Autodesk Inventor part; units mm, degrees
ref_plane "工作平面1" through (0, 0, 5.8) normal (0, 0, 1) x (1, 0, 0)
ref_plane "YZ Plane" through (0, 0, 0) normal (1, 0, 0) x (0, 1, 0)
ref_plane "XZ Plane" through (0, 0, 0) normal (0, 1, 0) x (-1, 0, 0)
sketch "草圖1" plane through (0, 0, 0) normal (0, 0, 1) x (1, 0, 0)
  circle A0 centre (0, 0) radius 26
  dimension "d0" = 52
extrude "擠出1" add sketch "草圖1" along normal blind 12.2
sketch "草圖2" plane through (0, 0, 12.2) normal (0, 0, 1) x (1, 0, 0)
  circle A0 centre (0, 0) radius 26
  circle A1 centre (0, 0) radius 20
  dimension "d3" = 40
extrude "擠出2" cut sketch "草圖2" against normal through all contours A1
sketch "草圖3" plane through (0, 0, 0) normal (0, 0, -1) x (-1, 0, 0)
  circle A0 centre (0, 0) radius 20
  circle A1 centre (0, 0) radius 26
  circle A2 centre (0, 0) radius 22.45
  dimension "d6" = 44.9
extrude "擠出3" cut sketch "草圖3" against normal blind 8.2 contours A2
ref_plane "工作平面1" through (0, 0, 5.8) normal (0, 0, 1) x (1, 0, 0)
sketch "草圖4" plane through (0, 0, 5.8) normal (0, 0, 1) x (1, 0, 0)
  circle A0 centre (0, 0) radius 24.4
  circle A1 centre (0, 0) radius 26
  dimension "d10" = 48.8
extrude "擠出4" cut sketch "草圖4" against normal blind 2.8
chamfer "倒角1" distance 0.4 angle 45 3 edges at (-26, 0, 12.2) (-26, 0, 0) (22.45, 0, 0)
chamfer "倒角2" distance 0.3 angle 45 2 edges at (-20, 0, 8.2) (-20, 0, 12.2)
properties part number "鑄鐵SLEEVE"
Check sheet for the modelled part. Datum: model origin and axes. Units: mm. A direction names the side the tool comes from. Round coordinates to 2 decimals unless told otherwise and drop trailing zeros. Write each loop counter-clockwise with the first axis right and the second up, starting at its lowest first coordinate (ties: lowest second). Pieces come first, ordered by that corner, then holes. Notation, with made-up numbers: (73.5, 86.25) -> (98.5, 86.25) arc R14 cw to (98.5, 92.25) -> close; hole circle Ø3 at (69.5, -38). An arc over 180 degrees is marked (long way). Put each result on its own line as item: value.
(1) Tool access check on faces 1 (the face through (-4.336, -19.524, 10.224)), 2 (the face through (-24.376, 1.073, 4.42)). Record the directions out of +Z, -Z, +X, -X, +Y, -Y that give a thin tool (end or side, any length) a straight path to the whole face; none if there is none.
Values found:
face 1: +Z, -Z
face 2: none
(2) Sectioned sample at D-D (z = 10.5). Enter the section's corners in (x, y).
Values found:
outline: circle Ø52 at (0, 0); hole circle Ø40 at (0, 0)
(3) Go/stop test with flat-tipped pins: pin 1 Ø10 at (x, y) = (6.5, -20.5) entering from -Z; pin 2 Ø4 at (x, z) = (-14.5, 9.5) entering from -Y; pin 3 Ø1 at (x, z) = (-11, 8) entering from -Y; pin 4 Ø6 at (y, z) = (-10, 6) entering from -X. Record where each tip stops, or that it passes through.
Values found:
pin 1: stops at z = 0
pin 2: stops at y = -22.8
pin 3: stops at y = -23.79
pin 4: stops at x = -25.04
(4) Mould release check, pull along X, two halves, no side actions. Record for faces 3 (the face through (17, -12, 8.2)), 4 (the face through (-20.633, 15.821, 8.758)), 5 (the face through (-15.3, 17.2, 0)), 6 (the face through (16.55, 15.17, 4.25)): released by +X, released by -X, zero draft, split by the parting line, or undercut.
Values found:
face 3: undercut
face 4: split by the parting line
face 5: zero draft
face 6: undercut
(5) Sectioned sample at C-C (z = 3.75). Enter the section's corners in (x, y), plus the area to 3 significant figures.
Values found:
outline: circle Ø48.8 at (0, 0); hole circle Ø44.9 at (0, 0)
area: 287 mm^2
(6) Material ranges on line 1 (Z direction, x = 21, y = 14); line 2 (Y direction, x = 0, z = 3.25); line 3 (Z direction, x = -7.5, y = -21), recorded low to high.
Values found:
line 1: z = 0 to 3, 5.8 to 12.2
line 2: y = -24.4 to -22.45, 22.45 to 24.4
line 3: z = 8.2 to 12.2
